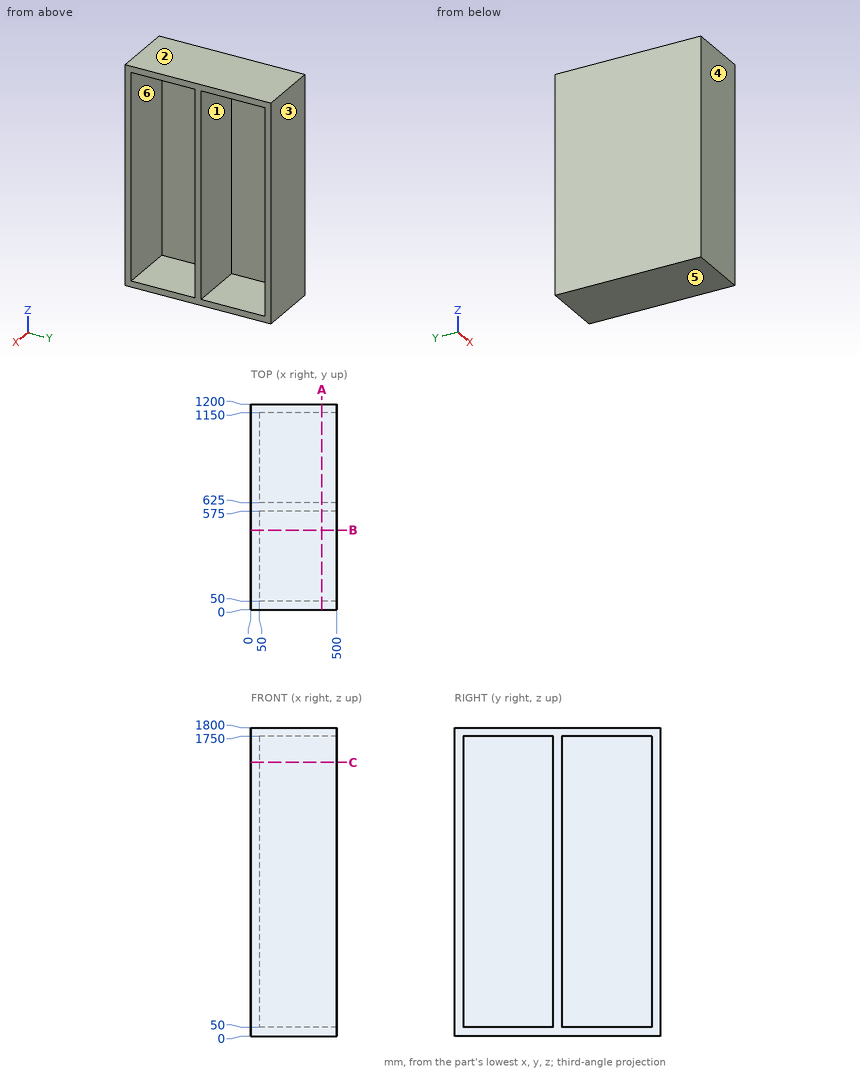
Study the drawing (mm; zero at the part's minimum x, y, z) and answer. A direction names the side the tool comes from. Coordinates: 2 decimals unless noted, no trailing zeros. Loops run counter-clockwise (first coordinate to the right, second up) from the corner with the lowest first, then second, coordinate; pieces in that order, holes last. Notation, with made-up numbers: M -1,-31.75 L 21,-31.75 A9 ccw 21,-22.75 Z; hole C 29,70 d3. An arc over 180 degrees is marked long. Answer as a JSON object with one key per item and string values. Group by question number.
Item 1: Determine the mould class of the marked faces 3, 4, 5 and 6 for opening direction Y: +Y half, -Y half, draft (parallel to the pull), parting line (faces both ways), or undercut.
Item 2: Which of the six approach directions +Z, -Z, +X, -X, +Y, -Y give full straight-line access (tool end or side, diameter ignored) to the marked faces 1 and 2?
Item 3: Section C-C (z = 1597) is taken. Write down the section's boundary in (x, y).
Item 4: Consider L1, parallel to Y at x = 460, z = 957; L2, parallel to Z at x = 463.5, y = 233.5; L3, parallel to X at y = 1061, z = 1700. Determine where each line is inside the solid, lowest interval first.
Item 5: Section A-A (x = 414) is taken. Write down the section's boundary in (y, z).
Item 6: Each of these flat-tipped pins is pushed along its axis until it touches: P1, Ø5, axis at y = 613.5, z = 1216, coming from the -X side; P2, Ø1.5, axis at y = 125, z = 1403, coming from the +X side. Where does it stop, or does it pass through?
Item 7: Section B-B (y = 464.5) is taken. Write down the section's boundary in (x, z), and give its area (3 significant figures).
Solved:
{
 "1": {"face 3": "+Y half", "face 4": "-Y half", "face 5": "draft", "face 6": "undercut"},
 "2": {"face 1": "+X", "face 2": "+Z, +X, -X, +Y, -Y"},
 "3": {"outline": "M 0,0 L 500,0 L 500,50 L 50,50 L 50,575 L 500,575 L 500,625 L 50,625 L 50,1150 L 500,1150 L 500,1200 L 0,1200 Z"},
 "4": {"L1": "y = 0 to 50, 575 to 625, 1150 to 1200", "L2": "z = 0 to 50, 1750 to 1800", "L3": "x = 0 to 50"},
 "5": {"outline": "M 0,0 L 1200,0 L 1200,1800 L 0,1800 Z; hole M 50,50 L 575,50 L 575,1750 L 50,1750 Z; hole M 625,50 L 1150,50 L 1150,1750 L 625,1750 Z"},
 "6": {"P1": "stops at x = 0", "P2": "stops at x = 50"},
 "7": {"outline": "M 0,0 L 500,0 L 500,50 L 50,50 L 50,1750 L 500,1750 L 500,1800 L 0,1800 Z", "area": "135,000 mm2"}
}
